Could you check a few things on this model? Use its own coordinates, in mm. Face numbers are marked on the shaded views. A direction names the side the tool comes from. Round coordinates to 2 decimals unless told otherwise and drop trailing zeros. Write each loop counter-clockwise with the first axis right and the second up, starting at its lowest first coordinate (ties: lowest second). Pieces come first, ordered by that corner, then holes. Notation, with made-up numbers: (24.25, 18.5) - (42.25, 18.5) arc R24 cw to (42.25, 33.5) - close; hole circle Ø5 at (33.25, 9.5). An arc over 180 degrees is marked (long way). Put each result on its own line as item: value.
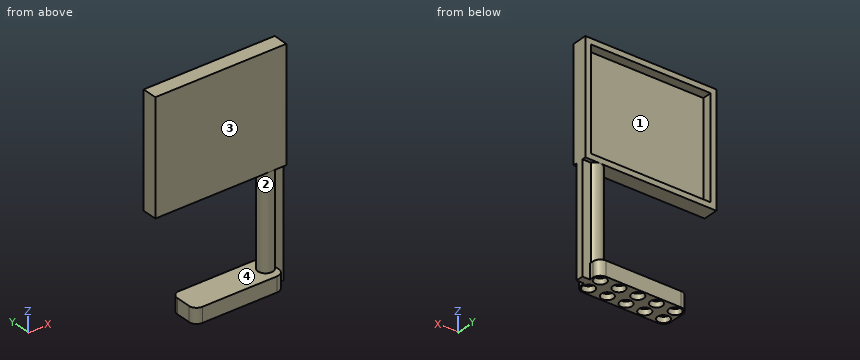
from build123d import *

# Parameters (mm, degrees)
EXTRUDE_1_DEPTH      = 5
EXTRUDE_1_DEPTH_BACK = 50
SKETCH_13_R          = 8.470611641
CUT_EXTRUDE_6_DEPTH  = 5
EXTRUDE_7_DEPTH      = 8
SKETCH_27_W          = 4
SKETCH_27_H          = 4
EXTRUDE_9_DEPTH      = 8
SKETCH_24_R          = 3.2
CUT_EXTRUDE_9_DEPTH  = 3.05
SKETCH_21_W          = 70
SKETCH_21_H          = 8
EXTRUDE_6_DEPTH      = 60
SKETCH_22_W          = 64
SKETCH_22_H          = 54
CUT_EXTRUDE_8_DEPTH  = 5


with BuildPart() as part:
    # ｽｹｯﾁ1 → ﾎﾞｽ - 押し出し1 (new, two sides: drawn at the far end of the back side and taken through both)
    with BuildSketch(Plane.XY.offset(-EXTRUDE_1_DEPTH_BACK)):
        with BuildLine():
            Line((3.464101615, 2), (8, 2))
            Line((8, 2), (8, -2))
            Line((8, -2), (3.464101615, -2))
            ThreePointArc((3.464101615, -2), (-4, 0), (3.464101615, 2))
        make_face()
    extrude(amount=EXTRUDE_1_DEPTH + EXTRUDE_1_DEPTH_BACK)

    # ｽｹｯﾁ13 → ｶｯﾄ - 押し出し6 (cut)
    with BuildSketch(Plane.XY.offset(5)):
        Circle(SKETCH_13_R)
    extrude(amount=-CUT_EXTRUDE_6_DEPTH, mode=Mode.SUBTRACT)

    # ｽｹｯﾁ23 → ﾎﾞｽ - 押し出し7 (add)
    with BuildSketch(Plane(origin=(0, 0, -50), x_dir=(-1, 0, 0), z_dir=(0, 0, -1))):
        with BuildLine():
            Line((-4, 4), (-4, -4))
            ThreePointArc((-4, -4), (-2.828427125, -6.828427125), (0, -8))
            Line((0, -8), (40, -8))
            ThreePointArc((40, -8), (42.828427125, -6.828427125), (44, -4))
            Line((44, -4), (44, 4))
            ThreePointArc((44, 4), (42.828427125, 6.828427125), (40, 8))
            Line((40, 8), (0, 8))
            ThreePointArc((0, 8), (-2.828427125, 6.828427125), (-4, 4))
        make_face()
    extrude(amount=EXTRUDE_7_DEPTH)

    # ｽｹｯﾁ27 → ﾎﾞｽ - 押し出し9 (add)
    with BuildSketch(Plane(origin=(0, 0, -50), x_dir=(-1, 0, 0), z_dir=(0, 0, -1))):
        with Locations((-6, 0)):
            Rectangle(SKETCH_27_W, SKETCH_27_H)
    extrude(amount=EXTRUDE_9_DEPTH)

    # ｽｹｯﾁ24 → ｶｯﾄ - 押し出し9 (cut)
    with BuildSketch(Plane(origin=(0, 0, -58), x_dir=(-1, 0, 0), z_dir=(0, 0, -1))):
        with Locations((0, 4)):
            Circle(SKETCH_24_R)
        with Locations((40, 4)):
            Circle(SKETCH_24_R)
        with Locations((40, -4)):
            Circle(SKETCH_24_R)
        with Locations((0, -4)):
            Circle(SKETCH_24_R)
        with Locations((10, 4)):
            Circle(SKETCH_24_R)
        with Locations((20, 4)):
            Circle(SKETCH_24_R)
        with Locations((30, 4)):
            Circle(SKETCH_24_R)
        with Locations((10, -4)):
            Circle(SKETCH_24_R)
        with Locations((20, -4)):
            Circle(SKETCH_24_R)
        with Locations((30, -4)):
            Circle(SKETCH_24_R)
    extrude(amount=-CUT_EXTRUDE_9_DEPTH, mode=Mode.SUBTRACT)

    # ｽｹｯﾁ21 → ﾎﾞｽ - 押し出し6 (add)
    with BuildSketch(Plane.XY):
        with Locations((-27, 0)):
            Rectangle(SKETCH_21_W, SKETCH_21_H)
    extrude(amount=EXTRUDE_6_DEPTH)

    # ｽｹｯﾁ22 → ｶｯﾄ - 押し出し8 (cut)
    with BuildSketch(Plane(origin=(0, 4, 0), x_dir=(1, 0, 0), z_dir=(0, 1, 0))):
        with Locations((-27, -30)):
            Rectangle(SKETCH_22_W, SKETCH_22_H)
    extrude(amount=-CUT_EXTRUDE_8_DEPTH, mode=Mode.SUBTRACT)


solid = part.part
(1) Imagine slicing it at A-A, the plane x = -31. List the corners of the cut face in (y, z) for me, then the cut area to 3 significant figures.
Values found:
outline: (-8, -58) - (-7.04, -58) - (-7.04, -54.95) - (-0.96, -54.95) - (-0.96, -58) - (0.96, -58) - (0.96, -54.95) - (7.04, -54.95) - (7.04, -58) - (8, -58) - (8, -50) - (-8, -50) - close; (-4, 0) - (4, 0) - (4, 3) - (-1, 3) - (-1, 57) - (4, 57) - (4, 60) - (-4, 60) - close
area: 301 mm^2
(2) Please list where these lines run through material, in increasing order: probe 1 along Z at (x, y) = (-23, 2.25); probe 2 along Z at (x, y) = (-10, 2.5); probe 3 along Y at (x, z) = (-30, -56). Write a range as from..to.
Values found:
probe 1: z = -58..-50, 0..3, 57..60
probe 2: z = -54.95..-50, 0..3, 57..60
probe 3: y = -8..-7.2, -0.8..0.8, 7.2..8
(3) If we mould it in two halves opening along Z, with no side actions, what happens to the marked faces 3 and 4? For each: pulls with the +Z half, pulls with the -Z half, needs draft (parallel to the pull), parting line crosses it, or undercut.
Values found:
face 3: needs draft
face 4: undercut
(4) Imagine slicing it at D-D, the plane x = -20. List the corners of the cut face in (y, z) for me, then the cut area to 3 significant figures.
Values found:
outline: (-8, -58) - (-7.2, -58) - (-7.2, -54.95) - (-0.8, -54.95) - (-0.8, -58) - (0.8, -58) - (0.8, -54.95) - (7.2, -54.95) - (7.2, -58) - (8, -58) - (8, -50) - (-8, -50) - close; (-4, 0) - (4, 0) - (4, 3) - (-1, 3) - (-1, 57) - (4, 57) - (4, 60) - (-4, 60) - close
area: 299 mm^2
(5) I'm going to push flat-ended pins straight in: pin 1 (1.9 mm diameter, centred on x = -31.5, y = 5, fed in from -Z); pin 2 (3.5 mm diameter, centred on x = 5.5, z = -39.5, fed in from +Y); pin 3 (3.5 mm diameter, centred on x = 5.5, z = -20, fed in from -Y). Where does each tip first touch, or does it pass through?
Values found:
pin 1: stops at z = -54.95
pin 2: stops at y = 2
pin 3: stops at y = -2
(6) Imagine slicing it at C-C, the plane x = -48. List the corners of the cut face in (y, z) for me, then the cut area to 3 significant figures.
Values found:
outline: (-4, 0) - (4, 0) - (4, 3) - (-1, 3) - (-1, 57) - (4, 57) - (4, 60) - (-4, 60) - close
area: 210 mm^2
(7) For the marked faces 1 and 2, which set-ups out of +Z, -Z, +X, -X, +Y, -Y let a thin tool reach every point of the face, with its end or its side?
Values found:
face 1: +Y
face 2: none
(8) Imagine slicing it at B-B, the plane z = 44. List the corners of the cut face in (x, y) for me.
Values found:
outline: (-62, -4) - (8, -4) - (8, 4) - (5, 4) - (5, -1) - (-59, -1) - (-59, 4) - (-62, 4) - close
